The listing builds one solid part. Answer for the finished solid, in the listing's coordinates (mm). Round coordinates to 2 decimals unless told otherwise and drop trailing zeros. Order: outer loops, then holes, each group sorted by start corner. A loop starts at its lowest first (then second) coordinate and runs counter-clockwise, first axis right, second up. Notation, with made-up numbers: (47, 89.25) -> (100, 89.25) arc R16 ccw to (100, 97.25) -> close; hole circle Ø9 at (88, 28). An arc over 180 degrees is marked (long way). Answer in a Markdown table with one row per item. Add a question column.
```python
from build123d import *

# Parameters (mm, degrees)
SKETCH1_W           = 5.079991364
SKETCH1_H           = 107.95
BOSS_EXTRUDE1_DEPTH = 5.08
CUT_EXTRUDE1_REACH  = 103.848
SKETCH3_R           = 1.143


with BuildPart() as part:
    # Sketch1 → Boss-Extrude1 (new body)
    with BuildSketch(Plane.XY):
        with Locations((-0.039375527, -47.713604651)):
            Rectangle(SKETCH1_W, SKETCH1_H)
    extrude(amount=BOSS_EXTRUDE1_DEPTH)

    # Sketch3 → Cut-Extrude1 (cut, up to next)
    with BuildSketch(Plane.XY.offset(5.08), mode=Mode.PRIVATE) as cut_extrude1_sk1:
        with Locations((-0.039375527, -47.713604651)):
            Circle(SKETCH3_R)
    cut_extrude1_tool1 = extrude(cut_extrude1_sk1.sketch, amount=-CUT_EXTRUDE1_REACH, mode=Mode.PRIVATE) & part.part
    # Sketch3 → Cut-Extrude1 (cut, up to next)
    with BuildSketch(Plane.XY.offset(5.08), mode=Mode.PRIVATE) as cut_extrude1_sk2:
        with Locations((-0.039375527, 1.286395349)):
            Circle(SKETCH3_R)
    cut_extrude1_tool2 = extrude(cut_extrude1_sk2.sketch, amount=-CUT_EXTRUDE1_REACH, mode=Mode.PRIVATE) & part.part
    # Sketch3 → Cut-Extrude1 (cut, up to next)
    with BuildSketch(Plane.XY.offset(5.08), mode=Mode.PRIVATE) as cut_extrude1_sk3:
        with Locations((0, -96.713604651)):
            Circle(SKETCH3_R)
    cut_extrude1_tool3 = extrude(cut_extrude1_sk3.sketch, amount=-CUT_EXTRUDE1_REACH, mode=Mode.PRIVATE) & part.part
    add(cut_extrude1_tool1.solids().sort_by_distance((-0.039376, -47.713605, 5.08))[0], mode=Mode.SUBTRACT)
    add(cut_extrude1_tool2.solids().sort_by_distance((-0.039376, 1.286395, 5.08))[0], mode=Mode.SUBTRACT)
    add(cut_extrude1_tool3.solids().sort_by_distance((0, -96.713605, 5.08))[0], mode=Mode.SUBTRACT)


solid = part.part
```
1. The part is cut by section B-B (z = 3). Give the vertices of the cut face in (x, y), then the cut area to 3 significant figures.
2. The mould has two halves that part along Y. Classify faces 1 (the flat face through (2.501, -48, 3)), 2 (the cylindrical face through (-0.29, -48.83, 2.58)), 3 (the flat face through (0, 6.261, 3)): released by +Y, released by -Y, zero draft, split by the parting line, or undercut.
3. The part is cut by section A-A (x = -0.1). Give the vertices of the cut face in (y, z) (3 decimals).
4. Straight lines are drawn through the part: line 1 along Y through (x, z) = (0.05, 1.1); line 2 along Y through (x, z) = (-0.9, 3.85); line 3 along X through (y, z) = (0.5, 0.4). For each, find the intervals that lie inside material, in ascending order.
Report:
| question | item | result |
|---|---|---|
| 1 | outline | (-2.58, -101.69) -> (2.5, -101.69) -> (2.5, 6.26) -> (-2.58, 6.26) -> close; hole circle Ø2.29 at (-0.04, -47.71); hole circle Ø2.29 at (-0.04, 1.29); hole circle Ø2.29 at (0, -96.71) |
| 1 | area | 536 mm^2 |
| 2 | face 1 | zero draft |
| 2 | face 2 | undercut |
| 2 | face 3 | released by +Y |
| 3 | outline | (-101.689, 0) -> (-97.852, 0) -> (-97.852, 5.08) -> (-101.689, 5.08) -> close; (-95.575, 0) -> (-48.855, 0) -> (-48.855, 5.08) -> (-95.575, 5.08) -> close; (-46.572, 0) -> (0.145, 0) -> (0.145, 5.08) -> (-46.572, 5.08) -> close; (2.428, 0) -> (6.261, 0) -> (6.261, 5.08) -> (2.428, 5.08) -> close |
| 4 | line 1 | y = -101.69 to -97.86, -95.57 to -48.85, -46.57 to 0.15, 2.43 to 6.26 |
| 4 | line 2 | y = -101.69 to -97.42, -96.01 to -48.47, -46.96 to 0.53, 2.04 to 6.26 |
| 4 | line 3 | x = -2.58 to -0.87, 0.79 to 2.5 |
